from build123d import *

# Parameters (mm, degrees)
SKETCH1_R                = 38.1
CENTERHUB_DEPTH          = 20.6375
RIB_DEPTH                = 3.175
LIGHTENING_HOLE_DEPTH    = 21.6375
FILLET1_R                = 6.35
CIRPATTERN1_COUNT        = 6
FILLET1_OF_CIRPATTERN1_R = 6.35
SKETCH5_R                = 19.05
THRU_HOLE_DEPTH          = 21.6375
THRU_HOLE_DEPTH_BACK     = 21.6375


with BuildPart() as part:
    # Sketch1 → CenterHub (new body, symmetric)
    with BuildSketch(Plane.XY):
        Circle(SKETCH1_R)
    extrude(amount=CENTERHUB_DEPTH, both=True)

    # Sketch2 → Rim and Web (revolve)
    with BuildSketch(Plane(origin=(0, 0, 0), x_dir=(0, 0, -1), z_dir=(1, 0, 0))):
        Polygon((-6.35, 0), (6.35, 0), (6.35, 165.1), (19.05, 165.1), (19.05, 177.8), (-19.05, 177.8), (-19.05, 165.1), (-6.35, 165.1), align=None)
    revolve(axis=Axis((0, 0, 0), (0, 0, -1)))

    # Sketch3 → Rib (add, symmetric)
    with BuildSketch(Plane(origin=(0, 0, 0), x_dir=(1, 0, 0), z_dir=(0, 1, 0))):
        Polygon((0, -19.05), (132.747036773, -19.05), (167.64, -6.35), (167.64, 6.35), (132.747036773, 19.05), (0, 19.05), align=None)
    rib = extrude(amount=RIB_DEPTH, both=True)

    # Sketch4 → Lightening hole (cut, symmetric)
    with BuildSketch(Plane.XY):
        with BuildLine():
            Line((92.100127656, -121.422100483), (43.438552305, -37.1377796))
            ThreePointArc((43.438552305, -37.1377796), (49.493351826, -28.575), (53.881536726, -19.05))
            Line((53.881536726, -19.05), (151.204687427, -19.05))
            ThreePointArc((151.204687427, -19.05), (131.982271537, -76.2), (92.100127656, -121.422100483))
        make_face()
    lightening_hole = extrude(amount=LIGHTENING_HOLE_DEPTH, both=True, mode=Mode.SUBTRACT)

    # Fillet1
    fillet1_edges = [part.edges().sort_by_distance(p)[0] for p in [
        (151.204687427, -19.05, 0),
        (92.100127656, -121.422100483, 0),
        (43.438552305, -37.1377796, 0),
        (53.881536726, -19.05, 0),
    ]]
    fillet(fillet1_edges, radius=FILLET1_R)

    # CirPattern1: Rib, Lightening hole ×6 about axis
    cirpattern1_axis = Axis((0, 0, 0), (0, 0, 1))
    for i in range(1, CIRPATTERN1_COUNT):
        add(rib.rotate(cirpattern1_axis, i * 360 / CIRPATTERN1_COUNT))
        add(lightening_hole.rotate(cirpattern1_axis, i * 360 / CIRPATTERN1_COUNT), mode=Mode.SUBTRACT)

    # Fillet1 of CirPattern1
    fillet1_of_cirpattern1_edges = [part.edges().sort_by_distance(p)[0] for p in [
        (92.100127656, 121.422100483, 0),
        (151.204687427, 19.05, 0),
        (53.881536726, 19.05, 0),
        (43.438552305, 37.1377796, 0),
        (-59.104559772, 140.472100483, 0),
        (59.104559772, 140.472100483, 0),
        (10.442984421, 56.1877796, 0),
        (-10.442984421, 56.1877796, 0),
        (-151.204687427, 19.05, 0),
        (-92.100127656, 121.422100483, 0),
        (-43.438552305, 37.1377796, 0),
        (-53.881536726, 19.05, 0),
        (-92.100127656, -121.422100483, 0),
        (-151.204687427, -19.05, 0),
        (-53.881536726, -19.05, 0),
        (-43.438552305, -37.1377796, 0),
        (59.104559772, -140.472100483, 0),
        (-59.104559772, -140.472100483, 0),
        (-10.442984421, -56.1877796, 0),
        (10.442984421, -56.1877796, 0),
    ]]
    fillet(fillet1_of_cirpattern1_edges, radius=FILLET1_OF_CIRPATTERN1_R)

    # Sketch5 → Thru hole (cut, two sides)
    with BuildSketch(Plane.XY) as thru_hole_sk:
        Circle(SKETCH5_R)
    extrude(amount=THRU_HOLE_DEPTH, mode=Mode.SUBTRACT)
    extrude(thru_hole_sk.sketch, amount=-THRU_HOLE_DEPTH_BACK, mode=Mode.SUBTRACT)


solid = part.part
Design review of the part built by this model. Coordinates are the model's own, in mm. A direction names the side the tool comes from. Coordinates: 2 decimals unless noted, no trailing zeros. Order: outer loops, then holes, each group sorted by start corner. A loop starts at its lowest first (then second) coordinate and runs counter-clockwise, first axis right, second up. Notation, with made-up numbers: (41, 86) - (60, 86) arc R16 ccw to (60, 99) - close; hole circle Ø6 at (-12, 66). An arc over 180 degrees is marked (long way). Put each result on its own line as item: value.
1) Wall thickness on L1, parallel to X at y = -65, z = -16.5; L2, parallel to Y at x = 59.5, z = 1.5; L3, parallel to Y at x = -103.5, z = 8.5 (3 decimals): over which ranges is each line inside the solid? List them lowest first. Write a range as from..to.
Response values:
L1: x = -165.49..-151.77, -41.19..-33.86, 33.86..41.19, 151.77..165.49
L2: y = -167.55..-64.96, -19.05..19.05, 64.96..167.55
L3: y = -144.57..-128.63, -3.175..3.175, 128.63..144.57
2) Take a section at B-B, the plane x = 0. Count the separate pieces of the cut face and the enclosed holes in it, and give its area (3 significant figures).
Response values:
separate pieces: 4
enclosed holes: 0
area: 3,350 mm²
3) Tool access review of faces 3 (the face through (47.56, 88.73, 12.61)), 4 (the face through (47.56, 88.73, -12.79)), 5 (the face through (0.7, -152.4, 0.1)): name each direction out of +Z, -Z, +X, -X, +Y, -Y from which nothing blocks a thin tool from reaching the whole face with its end or side.
Response values:
face 3: +Z
face 4: -Z
face 5: +Z, -Z
4) The part is to be moulded in two halves that separate along X. For faces 1 (the face through (-157, 52, 19.05)), 2 (the face through (-47.56, 88.73, 12.61)), say which applies: released by +X, released by -X, zero draft, split by the parting line, or undercut.
Response values:
face 1: zero draft
face 2: undercut
5) Take a section at A-A, the plane z = 15. Give the boundary of the cut face in (x, y) (3 decimals).
Response values:
outline: circle Ø355.6 at (0, 0); (-143.874, -3.175) - (-37.967, -3.175) arc R38.1 ccw to (-21.733, -31.293) - (-74.687, -123.011) - (-69.188, -126.186) - (-16.234, -34.468) arc R38.1 ccw to (16.234, -34.468) - (69.188, -126.186) - (74.687, -123.011) - (21.733, -31.293) arc R38.1 ccw to (37.967, -3.175) - (143.874, -3.175) - (143.874, 3.175) - (37.967, 3.175) arc R38.1 ccw to (21.733, 31.293) - (74.687, 123.011) - (69.188, 126.186) - (16.234, 34.468) arc R38.1 ccw to (-16.234, 34.468) - (-69.188, 126.186) - (-74.687, 123.011) - (-21.733, 31.293) arc R38.1 ccw to (-37.967, 3.175) - (-143.874, 3.175) - close; hole circle Ø330.2 at (0, 0); hole circle Ø38.1 at (0, 0)
6) Insertion check: P1, Ø1, axis at y = 20.5, z = 5.5, coming from the -X side; P2, Ø8, axis at x = 86.5, z = 14.5, coming from the -Y side; P3, Ø14, axis at x = -77.5, z = 12.5, coming from the +Y side. Each pin has a flat end and moves straight along its axis. Give the tip position at first contact, or say it passes through.
Response values:
P1: stops at x = -176.67
P2: stops at y = -157.5
P3: stops at y = 163.23
